```python
from build123d import *

# Parameters (mm, degrees)
F0_W      = 50.8
F0_H      = 50.8
F0_W_2    = 31.75
F0_H_2    = 31.75
F1_DEPTH  = 15.875
F3_DEPTH  = 19.05
F5_DEPTH  = 25.4
F6_R      = 19.04999
F7_W      = 19.05
F7_H      = 12.7
F8_DEPTH  = 56.6950905122
F9_SIZE   = 9.525
F10_DEPTH = 38.101


# Not quite as in the source:
# - a fillet or chamfer is up to 0.001 mm smaller than in the source, because OpenCascade refuses the exact size


with BuildPart() as f1:
    # F0 (on Top) → F1 (new body, symmetric)
    with BuildSketch(Plane.XY):
        Rectangle(F0_W, F0_H)
        Rectangle(F0_W_2, F0_H_2, mode=Mode.SUBTRACT)
    extrude(amount=F1_DEPTH, both=True)

    # F2 (on Front) → F3 (join, symmetric)
    with BuildSketch(Plane.XZ):
        Polygon((-73.4620968847, -31.75), (-29.4680063725, -6.35), (34.0319936275, -6.35), (78.0260841398, 19.05), (71.6760841398, 30.0485226281), (30.6290388837, 6.35), (-32.8709611163, 6.35), (-79.8120968847, -20.7514773719), align=None)
    extrude(amount=F3_DEPTH, both=True)

    # F4 (on face) → F5 (cut)
    with BuildSketch(Plane(origin=(-10.9673709361, 0, 18.9960436868), x_dir=(0.8660254038, 0, 0.5), z_dir=(-0.5, 0, 0.8660254038))):
        with BuildLine():
            Line((-52.5075421174, 7.9375), (-60.4450421174, 7.9375))
            ThreePointArc((-60.4450421174, 7.9375), (-66.0577021931, 5.6126600757), (-68.3825421174, 0))
            ThreePointArc((-68.3825421174, 0), (-66.0577021931, -5.6126600757), (-60.4450421174, -7.9375))
            Line((-60.4450421174, -7.9375), (-52.5075421174, -7.9375))
            ThreePointArc((-52.5075421174, -7.9375), (-44.5700421174, 0), (-52.5075421174, 7.9375))
        make_face()
    extrude(amount=-F5_DEPTH, mode=Mode.SUBTRACT)

    # F6 (radius 19.05 in the source; OpenCascade refuses exactly that, so slightly less here)
    f6_edges = [f1.edges().sort_by_distance(p)[0] for p in [
        (-76.637097, -19.05, -26.250739),
        (-76.637097, 19.05, -26.250739),
    ]]
    fillet(f6_edges, radius=F6_R)

    # F7 (on face) → F8 (cut, through all)
    with BuildSketch(Plane(origin=(4.9076290639, 0, -8.5002628834), x_dir=(0.8660254038, 0, 0.5), z_dir=(-0.5, 0, 0.8660254038))):
        with Locations((54.8725710229, 0)):
            Rectangle(F7_W, F7_H)
    extrude(amount=-F8_DEPTH, mode=Mode.SUBTRACT)

    # F9
    f9_edges = [f1.edges().sort_by_distance(p)[0] for p in [
        (74.851084, 19.05, 24.549261),
        (74.851084, -19.05, 24.549261),
    ]]
    chamfer(f9_edges, length=F9_SIZE)

    # F10 (cut, through all): a face of the model
    f10_faces = [f1.faces().sort_by_distance(p)[0] for p in [
        (0, 0, 6.35),
    ]]
    extrude(f10_faces, amount=-F10_DEPTH, mode=Mode.SUBTRACT)


solid = f1.part
```
Here's how the part is built. I have some questions about the finished solid (model axes, mm). A direction names the side the tool comes from. Coordinates: 2 decimals unless noted, no trailing zeros. Order: outer loops, then holes, each group sorted by start corner. A loop starts at its lowest first (then second) coordinate and runs counter-clockwise, first axis right, second up.
Item 1: Which directions (+Z, -Z, +X, -X, +Y, -Y) give clear straight access to the entire face, cutting with the end or side of a thin tool? Please do faces 1 (the face through (55, -6.35, 13)), 2 (the face through (28, 0, 6.35)), 3 (the face through (-45, -19.05, -8)), 4 (the face through (47, -19.05, 10)), 5 (the face through (0, 15.875, 0)).
Response values:
face 1: none
face 2: +Z, +Y, -Y
face 3: +Z, -Z, -X, -Y
face 4: +Z, -Z, +X, -Y
face 5: +Z, -Z
Item 2: If we section it at A-A, the plane z = 10.5: List the corners of the cut face in (x, y) for me (3 decimals), then the cut area to 3 significant figures.
Response values:
outline: (-25.4, -25.4) - (25.4, -25.4) - (25.4, 25.4) - (-25.4, 25.4) - close; (37.817, -19.05) - (63.217, -19.05) - (63.217, -6.35) - (46.301, -6.35) - (46.301, 6.35) - (63.217, 6.35) - (63.217, 19.05) - (37.817, 19.05) - close; hole (-15.875, -15.875) - (15.875, -15.875) - (15.875, 15.875) - (-15.875, 15.875) - close
area: 2,330 mm2
Item 3: I'm going to push flat-ended pins straight in: pin 1 Ø3 at (x, y) = (28.5, 13.5) entering from +Z; pin 2 Ø6.5 at (x, z) = (-57, -12) entering from +Y; pin 3 Ø1.5 at (x, y) = (-58, 9) entering from +Z; pin 4 Ø6 at (x, z) = (-13, -17.5) entering from +Y. Where does each tip first touch, or does it pass through?
Response values:
pin 1: stops at z = 6.35
pin 2: stops at y = 19.05
pin 3: stops at z = -7.73
pin 4: stops at y = 25.4
Item 4: If we section it at C-C, the plane y = -22: List the corners of the cut face in (x, z) for me (3 decimals), then the cut area to 3 significant figures.
Response values:
outline: (-25.4, -15.875) - (25.4, -15.875) - (25.4, 15.875) - (-25.4, 15.875) - close
area: 1,610 mm2
Item 5: Thinking about a two-plate mould opening in X: for faces 6 (the face through (74.896, -0.133, 24.472)), 7 (the face through (25.4, 0, 7)), 8 (the face through (-27, 0, -6.35)), 9 (the face through (0, -25.4, 0)), which applies, pulls with the +X half, pulls with the -X half, needs draft (parallel to the pull), parting line crosses it, or undercut?
Response values:
face 6: pulls with the +X half
face 7: undercut
face 8: undercut
face 9: needs draft
Item 6: If we section it at B-B, the plane x = 9.5: List the corners of the cut face in (y, z) for me (3 decimals).
Response values:
outline: (-25.4, -15.875) - (-15.875, -15.875) - (-15.875, 15.875) - (-25.4, 15.875) - close; (15.875, -15.875) - (25.4, -15.875) - (25.4, 15.875) - (15.875, 15.875) - close
Item 7: If we section it at D-D, the plane x = 54: List the corners of the cut face in (y, z) for me, then the cut area to 3 significant figures.
Response values:
outline: (-19.05, 5.18) - (-6.35, 5.18) - (-6.35, 19.84) - (-19.05, 19.84) - close; (6.35, 5.18) - (19.05, 5.18) - (19.05, 19.84) - (6.35, 19.84) - close
area: 372 mm2
Item 8: I need wall thicknesses on probe 1 along X at (y, z) = (11, 10) (3 decimals); probe 2 along X at (y, z) = (-9, -12) (3 decimals); probe 3 along X at (y, z) = (21, 0). Which ranges of each line are inside material? Lowest first, please.
Response values:
probe 1: x = -25.4 to -15.875, 15.875 to 25.4, 36.951 to 62.351
probe 2: x = -64.654 to -39.254, -25.4 to -15.875, 15.875 to 25.4
probe 3: x = -25.4 to 25.4
